Geometry check sheet. Reference: drawing and pictorial views, mm from the part's lowest x, y, z. Coordinates: 2 decimals unless noted, no trailing zeros. Loops run counter-clockwise (first coordinate to the right, second up) from the corner with the lowest first, then second, coordinate; pieces in that order, holes last. Notation, with made-up numbers: (75.5, 8.25) - (83.5, 8.25) arc R21 ccw to (83.5, 47.25) - close; hole circle Ø9 at (-11, 11.25). An arc over 180 degrees is marked (long way). Write each question's results on one line, items separated by ' | '. Start each with the question number.
1. Cross-section at A-A (x = 51.5). Record the cut outline in (y, z).
2. Thickness scan on line 1 (Y direction, x = 59, z = 1.05) (1 decimal); line 2 (X direction, y = 23.75, z = 0.95); line 3 (Y direction, x = 22.5, z = 0.3). Record the ranges inside material, lowest first. Write a range as [from, to].
3. Cross-section at C-C (z = 1). Give the number of separate pieces and of enclosed holes in the cut face, and give its area (4 significant figures).
4. Cross-section at D-D (y = 2.5). Record the cut outline in (x, z), and give its area (3 significant figures).
5. Cross-section at B-B (y = 16). Record the cut outline in (x, z).
6. Gauge pin test, flat ends, axial feed: P1, Ø2.5, axis at x = 9, y = 10, coming from the -Z side; P2, Ø0.9, axis at x = 66.5, z = 2, coming from the -Y side; P3, Ø0.9, axis at y = 7, z = 1, coming from the -X side; P4, Ø3, axis at x = 10.5, y = 17.5, coming from the -Z side. Record the tip position at first contact, or that the pin passes through.
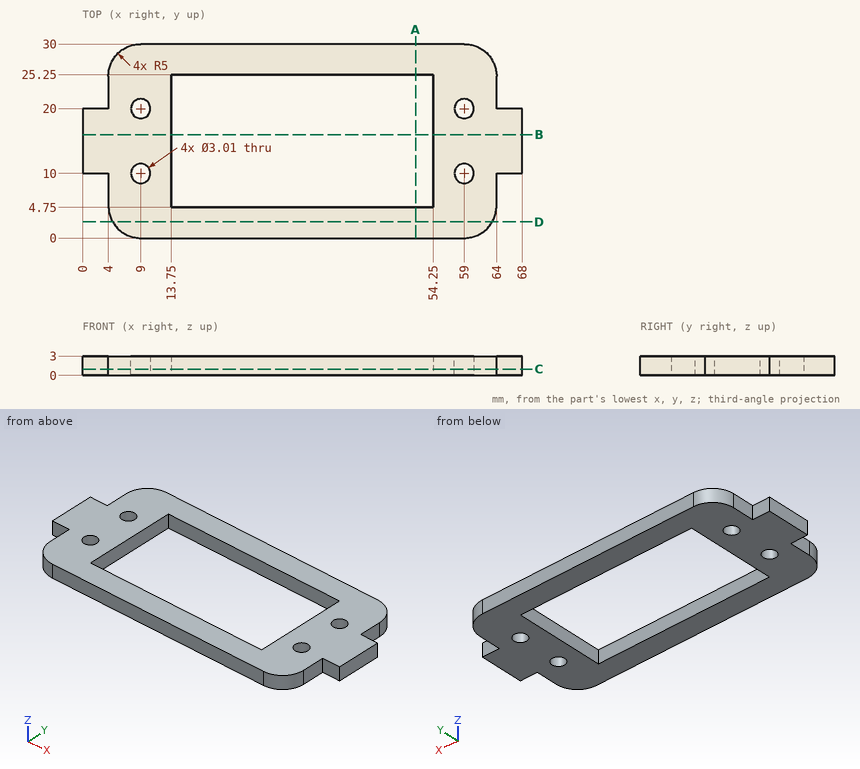
Established:
1) outline: (0, 0) - (4.75, 0) - (4.75, 3) - (0, 3) - close; (25.25, 0) - (30, 0) - (30, 3) - (25.25, 3) - close
2) line 1: [0, 8.5], [11.5, 18.5], [21.5, 30] | line 2: [4, 13.75], [54.25, 64] | line 3: [0, 4.75], [25.25, 30]
3) separate pieces: 1 | enclosed holes: 5 | area: 1,000 mm^2
4) outline: (4.67, 0) - (63.33, 0) - (63.33, 3) - (4.67, 3) - close | area: 176 mm^2
5) outline: (0, 0) - (13.75, 0) - (13.75, 3) - (0, 3) - close; (54.25, 0) - (68, 0) - (68, 3) - (54.25, 3) - close
6) P1: through | P2: y = 10 | P3: x = 4 | P4: z = 0
